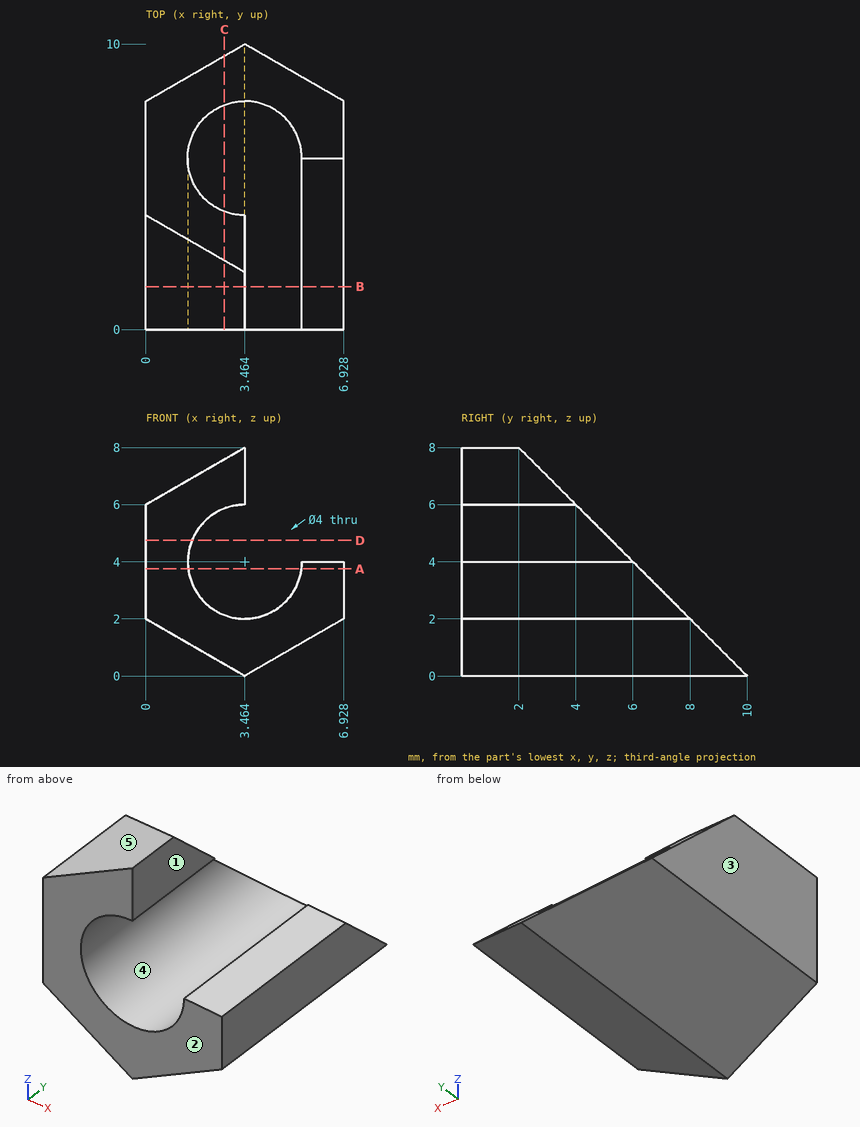
Design review of the part shown in the three views and the two pictorial views. Dimensions are in mm from the part's minimum x, y and z. A direction names the side the tool comes from. Round coordinates to 2 decimals unless told otherwise and drop trailing zeros. Loops run counter-clockwise (first coordinate to the right, second up) from the corner with the lowest first, then second, coordinate; pieces in that order, holes last. Notation, with made-up numbers: (47, -37) -> (69, -37) arc R15 cw to (69, -16) -> close; hole circle Ø2 at (14, -25). An arc over 180 degrees is marked (long way). Return JSON: item names as keys, results as strings.
(1) Add section A-A on z = 3.75. Write out the cut boundary in (x, y).
Solved:
{"outline": "(0, 0) -> (1.48, 0) -> (1.48, 6.25) -> (0, 6.25) -> close; (5.45, 0) -> (6.93, 0) -> (6.93, 6.25) -> (5.45, 6.25) -> close"}
(2) For line 1 (X direction, y = 1.5, z = 3); line 2 (Z direction, x = 2.75, y = 1); line 3 (Z direction, x = 2, y = 2.75) (1 decimal), list the stretches that pass through material, from the lowest coordinate up.
Solved:
{"line 1": "0 to 1.73, 5.2 to 6.93", "line 2": "0.41 to 2.13, 5.87 to 7.59", "line 3": "0.8 to 2.6, 5.4 to 7.2"}
(3) For pin 1 (3 mm diameter, centred on x = 4, z = 6.5, fed in from +Y); pin 2 (1 mm diameter, centred on y = 1.5, z = 6, fed in from +X); pin 3 (1.5 mm diameter, centred on x = 3, z = 2.5, fed in from +Y); pin 4 (2.5 mm diameter, centred on x = 3.46, z = 4, fed in from -Y), all flat-tipped, find the tip position at first contact; note any pin that passes through.
Solved:
{"pin 1": "y = 4.17", "pin 2": "x = 3.46", "pin 3": "y = 8.25", "pin 4": "through"}
(4) The part is to be moulded in two halves that separate along Z. For the marked faces 3, 4 and 5, say which applies: released by +Z, released by -Z, zero draft, split by the parting line, or undercut.
Solved:
{"face 3": "zero draft", "face 4": "undercut", "face 5": "released by +Z"}
(5) For the marked faces 1 and 2, list the 3-axis set-ups (+Z, -Z, +X, -X, +Y, -Y) from which the entire face can be reached by the end or side of a thin tool; tool diameter is ignored.
Solved:
{"face 1": "+Z, +X, +Y, -Y", "face 2": "+Z, -Z, +X, -X, -Y"}
(6) Add section C-C on x = 2.75. Write out the cut boundary in (y, z), plus the area to 3 significant figures.
Solved:
{"outline": "(0, 0.41) -> (9.59, 0.41) -> (7.87, 2.13) -> (0, 2.13) -> close; (0, 5.87) -> (4.13, 5.87) -> (2.41, 7.59) -> (0, 7.59) -> close", "area": "20.6 mm2"}
(7) Add section B-B on y = 1.5. Write out the cut boundary in (x, z).
Solved:
{"outline": "(0, 2) -> (3.46, 0) -> (6.93, 2) -> (6.93, 4) -> (5.46, 4) arc R2 cw (long way) to (3.46, 6) -> (3.46, 8) -> (0, 6) -> close"}
(8) Add section D-D on z = 4.75. Write out the cut boundary in (x, y).
Solved:
{"outline": "(0, 0) -> (1.61, 0) -> (1.61, 5.25) -> (0, 5.25) -> close"}
